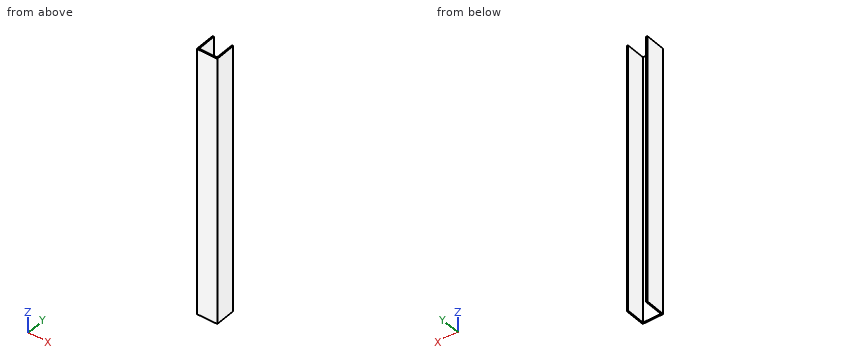
Autodesk Inventor part; units mm, degrees
ref_plane "YZ Plane" through (0, 0, 0) normal (1, 0, 0) x (0, 1, 0)
ref_plane "XZ Plane" through (0, 0, 0) normal (0, 1, 0) x (-1, 0, 0)
ref_plane "XY Plane" through (0, 0, 0) normal (0, 0, 1) x (1, 0, 0)
sketch "Sketch1" plane through (0, 0, 0) normal (0, 0, 1) x (1, 0, 0)
  line L0 (2.0066, 32.004) -> (0, 32.004)
  line L1 (0, 32.004) -> (0, 0)
  line L2 (0, 0) -> (2.0066, 0)
  line L3 (2.0066, 2.0066) -> (2.0066, 32.004)
  line L4 (2.0066, 0) -> (29.9974, 0)
  line L5 (29.9974, 2.0066) -> (2.0066, 2.0066)
  line L6 (29.9974, 0) -> (32.004, 0)
  line L7 (32.004, 0) -> (32.004, 32.004)
  line L8 (32.004, 32.004) -> (29.9974, 32.004)
  line L9 (29.9974, 32.004) -> (29.9974, 2.0066)
  dimension "d2" = 2.0066
  dimension "d3" = 32.004
sketch "Sketch2" plane through (0, 0, 0) normal (0, 0, 1) x (1, 0, 0)
  point P0 (0, 0)
extrude "Extrusion1" add sketch "Sketch1" along normal blind 418.846
properties part number "USEsolid7andsomething"
Input: part model. Units: mm. Frame: model coordinates. Give positions to 0.01 mm unless a question says otherwise; leave off trailing zeros. Write each loop counter-clockwise with the first axis right and the second up, starting at its lowest first coordinate (ties: lowest second). Pieces come first, ordered by that corner, then holes.
Q1. Section B-B, the plane z = 57. Output: boundary loops of the cut face in (x, y), plus the area to 3 significant figures.
Q2. Section C-C, the plane x = 11. Output: boundary loops of the cut face in (y, z).
Q3. Material intervals for probe 1 along X at (y, z) = (11, 377); probe 2 along Y at (x, z) = (12.5, 37), sorted ascending.
Q4. First-contact query: P1, Ø1.5, axis at x = 6.5, z = 303.5, coming from the +Y side. Flat tip, straight axial feed; report the tip coordinate or a pass-through.
Q5. Section A-A, the plane y = 9. Output: boundary loops of the cut face in (x, z).
Filled in:
1. outline: (0, 0) - (32, 0) - (32, 32) - (30, 32) - (30, 2.01) - (2.01, 2.01) - (2.01, 32) - (0, 32) - close
1. area: 185 mm2
2. outline: (0, 0) - (2.01, 0) - (2.01, 418.85) - (0, 418.85) - close
3. probe 1: x = 0 to 2.01, 30 to 32
3. probe 2: y = 0 to 2.01
4. P1: stops at y = 2.01
5. outline: (0, 0) - (2.01, 0) - (2.01, 418.85) - (0, 418.85) - close; (30, 0) - (32, 0) - (32, 418.85) - (30, 418.85) - close
